```python
from build123d import *

# Parameters (mm, degrees)
SKETCH1_W                     = 472
SKETCH1_H                     = 1
BASE_FLANGE1_DEPTH            = 590
EDGE_FLANGE1_STRIP_W          = 6
EDGE_FLANGE1_STRIP_H          = 1
EDGE_FLANGE1_STRIP_CUT_DEPTH  = 432
EDGE_FLANGE1_RELIEF_W         = 6.5
EDGE_FLANGE1_RELIEF_H         = 0.5
EDGE_FLANGE1_RELIEF_CUT_DEPTH = 1
EDGE_FLANGE1_DEPTH            = 432
EDGE_FLANGE2_STRIP_W          = 6
EDGE_FLANGE2_STRIP_H          = 1
EDGE_FLANGE2_STRIP_CUT_DEPTH  = 1140
EDGE_FLANGE2_RELIEF_W         = 6.5
EDGE_FLANGE2_RELIEF_H         = 0.5
EDGE_FLANGE2_RELIEF_CUT_DEPTH = 1
EDGE_FLANGE2_DEPTH            = 1140
SKETCH16_R                    = 3
CUT_EXTRUDE1_DEPTH            = 756.860436853
SKETCH18_R                    = 3
CUT_EXTRUDE2_DEPTH            = 1204.551826886


# Sheet-metal steps are written as plain solids
with BuildPart() as part:
    # Sketch1 → Base-Flange1 (new, symmetric)
    with BuildSketch(Plane(origin=(0, 0, 0), x_dir=(1, 0, 0), z_dir=(0, 1, 0))):
        with Locations((0, -0.5)):
            Rectangle(SKETCH1_W, SKETCH1_H)
    extrude(amount=BASE_FLANGE1_DEPTH, both=True)

    # Edge-Flange1 strip (across the edge) → Edge-Flange1 strip cut (cut)
    with BuildSketch(Plane(origin=(-216, -590, 1), x_dir=(0, 1, 0), z_dir=(1, 0, 0))):
        with Locations((-1, -0.5)):
            Rectangle(EDGE_FLANGE1_STRIP_W, EDGE_FLANGE1_STRIP_H)
    edge_flange1_strip_cut = extrude(amount=EDGE_FLANGE1_STRIP_CUT_DEPTH, mode=Mode.SUBTRACT)

    # Edge-Flange1 relief (on the sheet) → Edge-Flange1 relief cut (cut)
    with BuildSketch(Plane(origin=(-216, -588, 1), x_dir=(0, 1, 0), z_dir=(0, 0, 1))):
        with Locations((-2.75, 0.25)):
            Rectangle(EDGE_FLANGE1_RELIEF_W, EDGE_FLANGE1_RELIEF_H)
        with Locations((-2.75, -432.25)):
            Rectangle(EDGE_FLANGE1_RELIEF_W, EDGE_FLANGE1_RELIEF_H)
    edge_flange1_relief_cut = extrude(amount=-EDGE_FLANGE1_RELIEF_CUT_DEPTH, mode=Mode.SUBTRACT)

    # Edge-Flange1 section (across the edge) → Edge-Flange1 (add)
    with BuildSketch(Plane(origin=(-216, -590, 1), x_dir=(0, 1, 0), z_dir=(1, 0, 0))):
        with BuildLine():
            Line((0, 1), (0, 20))
            Line((0, 20), (1, 20))
            Line((1, 20), (1, 1))
            ThreePointArc((1, 1), (1.292893219, 0.292893219), (2, 0))
            Line((2, 0), (2, -1))
            ThreePointArc((2, -1), (0.585786438, -0.414213562), (0, 1))
        make_face()
    edge_flange1 = extrude(amount=EDGE_FLANGE1_DEPTH)

    # Mirror1: Edge-Flange1 strip cut, Edge-Flange1 relief cut, Edge-Flange1 across plane
    add(edge_flange1_strip_cut.mirror(Plane.ZX), mode=Mode.SUBTRACT)
    add(edge_flange1_relief_cut.mirror(Plane.ZX), mode=Mode.SUBTRACT)
    add(edge_flange1.mirror(Plane.ZX))

    # Edge-Flange2 strip (across the edge) → Edge-Flange2 strip cut (cut)
    with BuildSketch(Plane(origin=(-236, 570, 1), x_dir=(1, 0, 0), z_dir=(0, -1, 0))):
        with Locations((-1, -0.5)):
            Rectangle(EDGE_FLANGE2_STRIP_W, EDGE_FLANGE2_STRIP_H)
    edge_flange2_strip_cut = extrude(amount=EDGE_FLANGE2_STRIP_CUT_DEPTH, mode=Mode.SUBTRACT)

    # Edge-Flange2 relief (on the sheet) → Edge-Flange2 relief cut (cut)
    with BuildSketch(Plane(origin=(-234, 570, 1), x_dir=(1, 0, 0), z_dir=(0, 0, 1))):
        with Locations((-2.75, 0.25)):
            Rectangle(EDGE_FLANGE2_RELIEF_W, EDGE_FLANGE2_RELIEF_H)
        with Locations((-2.75, -1140.25)):
            Rectangle(EDGE_FLANGE2_RELIEF_W, EDGE_FLANGE2_RELIEF_H)
    edge_flange2_relief_cut = extrude(amount=-EDGE_FLANGE2_RELIEF_CUT_DEPTH, mode=Mode.SUBTRACT)

    # Edge-Flange2 section (across the edge) → Edge-Flange2 (add)
    with BuildSketch(Plane(origin=(-236, 570, 1), x_dir=(1, 0, 0), z_dir=(0, -1, 0))):
        with BuildLine():
            Line((0, 1), (0, 20))
            Line((0, 20), (1, 20))
            Line((1, 20), (1, 1))
            ThreePointArc((1, 1), (1.292893219, 0.292893219), (2, 0))
            Line((2, 0), (2, -1))
            ThreePointArc((2, -1), (0.585786438, -0.414213562), (0, 1))
        make_face()
    edge_flange2 = extrude(amount=EDGE_FLANGE2_DEPTH)

    # Mirror2: Edge-Flange2 strip cut, Edge-Flange2 relief cut, Edge-Flange2 across plane
    add(edge_flange2_strip_cut.mirror(Plane(origin=(0, 0, 0), x_dir=(0, 0, 1), z_dir=(1, 0, 0))), mode=Mode.SUBTRACT)
    add(edge_flange2_relief_cut.mirror(Plane(origin=(0, 0, 0), x_dir=(0, 0, 1), z_dir=(1, 0, 0))), mode=Mode.SUBTRACT)
    add(edge_flange2.mirror(Plane(origin=(0, 0, 0), x_dir=(0, 0, 1), z_dir=(1, 0, 0))))

    # Sketch16 → Cut-Extrude1 (cut, through all)
    with BuildSketch(Plane.ZY.offset(236)):
        with Locations((11.5, 520)):
            Circle(SKETCH16_R)
        with Locations((11.5, 320)):
            Circle(SKETCH16_R)
        with Locations((11.5, 120)):
            Circle(SKETCH16_R)
        with Locations(Location((11.5, -120, 0), (0, 0, 180))):
            Circle(SKETCH16_R)
        with Locations(Location((11.5, -320, 0), (0, 0, 180))):
            Circle(SKETCH16_R)
        with Locations(Location((11.5, -520, 0), (0, 0, 180))):
            Circle(SKETCH16_R)
    extrude(amount=-CUT_EXTRUDE1_DEPTH, mode=Mode.SUBTRACT)

    # Sketch18 → Cut-Extrude2 (cut, through all)
    with BuildSketch(Plane(origin=(0, 590, 0), x_dir=(1, 0, 0), z_dir=(0, 1, 0))):
        with Locations(Location((-181, -11.5, 0), (0, 0, 270))):
            Circle(SKETCH18_R)
        with Locations(Location((0, -11.5, 0), (0, 0, 270))):
            Circle(SKETCH18_R)
        with Locations(Location((181, -11.5, 0), (0, 0, 90))):
            Circle(SKETCH18_R)
    extrude(amount=-CUT_EXTRUDE2_DEPTH, mode=Mode.SUBTRACT)


solid = part.part
```
CAD build for the part. Positions are in the model's coordinates, mm. Round coordinates to 2 decimals unless told otherwise and drop trailing zeros. Write each loop counter-clockwise with the first axis right and the second up, starting at its lowest first coordinate (ties: lowest second). Pieces come first, ordered by that corner, then holes.
Item 1: Drop flat-ended pins along their axis: pin 1 Ø5 at (x, y) = (152, 342) entering from +Z; pin 2 Ø3 at (y, z) = (-589.5, 8) entering from +X; pin 3 Ø2 at (x, z) = (234.5, 15.5) entering from -Y. Give the stop position or say it passes through.
Filled in:
pin 1: stops at z = 1
pin 2: stops at x = 216
pin 3: stops at y = -570
Item 2: Band-saw the part on A-A on x = 128. Write the cut outline in (y, z), then the cut area to 3 significant figures.
Filled in:
outline: (-590, 2) arc R2 ccw to (-588, 0) - (588, 0) arc R2 ccw to (590, 2) - (590, 21) - (589, 21) - (589, 2) arc R1 cw to (588, 1) - (-588, 1) arc R1 cw to (-589, 2) - (-589, 21) - (-590, 21) - close
area: 1,220 mm2
Item 3: Mould opens along X. For faces 1 (the flat face through (-3, 8, 1)), 2 (the flat face through (-3, 8, 0)) say: released by +X, released by -X, zero draft, split by the parting line, or undercut.
Filled in:
face 1: undercut
face 2: zero draft
Item 4: Band-saw the part on B-B on y = -436. Write the cut outline in (x, z).
Filled in:
outline: (-236, 2) arc R2 ccw to (-234, 0) - (234, 0) arc R2 ccw to (236, 2) - (236, 21) - (235, 21) - (235, 2) arc R1 cw to (234, 1) - (-234, 1) arc R1 cw to (-235, 2) - (-235, 21) - (-236, 21) - close
Item 5: Drill centre lines: L1, parallel to X at y = 206, z = 19.25; L2, parallel to X at y = 589.55, z = 11.5; L3, parallel to Y at x = -113, z = 4. Where is each one in solid material? Low to high.
Filled in:
L1: x = -236 to -235, 235 to 236
L2: x = -216 to -184, -178 to -3, 3 to 178, 184 to 216
L3: y = -590 to -589, 589 to 590
